from build123d import *

# Parameters (mm, degrees)
SKETCH2_W           = 889
SKETCH2_H           = 860.425
SKETCH2_W_2         = 698.5
SKETCH2_H_2         = 685.8
BOSS_EXTRUDE1_DEPTH = 114.3
SKETCH3_W           = 82.55
SKETCH3_H           = 79.375
CUT_EXTRUDE1_DEPTH  = 115.3
FILLET1_R           = 6.35


with BuildPart() as part:
    # Sketch2 → Boss-Extrude1 (new body)
    with BuildSketch(Plane(origin=(0, 0, 0), x_dir=(1, 0, 0), z_dir=(0, 1, 0))):
        with Locations((0, 7.9375)):
            Rectangle(SKETCH2_W, SKETCH2_H)
        Rectangle(SKETCH2_W_2, SKETCH2_H_2, mode=Mode.SUBTRACT)
    extrude(amount=BOSS_EXTRUDE1_DEPTH)

    # Sketch3 → Cut-Extrude1 (cut, through all)
    with BuildSketch(Plane(origin=(0, 114.3, 0), x_dir=(1, 0, 0), z_dir=(0, 1, 0))):
        with Locations((168.275, -382.5875)):
            Rectangle(SKETCH3_W, SKETCH3_H)
    extrude(amount=-CUT_EXTRUDE1_DEPTH, mode=Mode.SUBTRACT)

    # Fillet1
    fillet1_edges = [part.edges().sort_by_distance(p)[0] for p in [
        (444.5, 114.3, -7.9375),
        (0, 114.3, -438.15),
        (327.025, 0, 422.275),
        (327.025, 114.3, 422.275),
        (-444.5, 114.3, -7.9375),
        (0, 0, -438.15),
        (444.5, 0, -7.9375),
        (-158.75, 0, 422.275),
        (-444.5, 0, -7.9375),
        (-444.5, 57.15, -438.15),
        (444.5, 57.15, -438.15),
        (444.5, 57.15, 422.275),
        (-444.5, 57.15, 422.275),
        (-158.75, 114.3, 422.275),
    ]]
    fillet(fillet1_edges, radius=FILLET1_R)


solid = part.part
Check sheet for the modelled part. Datum: model origin and axes. Units: mm. A direction names the side the tool comes from. Coordinates: 2 decimals unless noted, no trailing zeros. Write each loop counter-clockwise with the first axis right and the second up, starting at its lowest first coordinate (ties: lowest second). Pieces come first, ordered by that corner, then holes.
Item 1: Mould release check, pull along Z, two halves, no side actions. Record for faces 1 (the face through (349.25, 56, 5)), 2 (the face through (-6, 114.3, -391)), 3 (the face through (-160, 56, 422.275)), 4 (the face through (-6, 56, -438.15)): released by +Z, released by -Z, zero draft, split by the parting line, or undercut.
Numbers:
face 1: undercut
face 2: zero draft
face 3: released by +Z
face 4: released by -Z
Item 2: Access from +Z, -Z, +X, -X, +Y, -Y to the whole of each face (thin tool, end or side, straight path). Record for faces 5 (the face through (-6, 0, -391)), 6 (the face through (209.55, 58, 383)), 7 (the face through (-5, 56, -342.9)).
Numbers:
face 5: +Z, -Z, +X, -X, -Y
face 6: +Z, +Y, -Y
face 7: +Y, -Y
Item 3: Cross-section at B-B on x = -151.5. Record the boundary of the cut face in (y, z) (3 decimals).
Numbers:
outline: (0, -431.8) arc R6.35 ccw to (6.35, -438.15) - (107.95, -438.15) arc R6.35 ccw to (114.3, -431.8) - (114.3, -342.9) - (0, -342.9) - close; (0, 342.9) - (114.3, 342.9) - (114.3, 415.925) arc R6.35 ccw to (107.95, 422.275) - (6.35, 422.275) arc R6.35 ccw to (0, 415.925) - close
Item 4: Scan lines: probe 1 along X at (y, z) = (48.5, 306); probe 2 along X at (y, z) = (25, 357); probe 3 along Z at (x, y) = (-193.5, 46.5) (3 decimals). Record each from-to range of solid material in increasing order.
Numbers:
probe 1: x = -444.5 to -349.25, 349.25 to 444.5
probe 2: x = -444.5 to 127, 209.55 to 444.5
probe 3: z = -438.15 to -342.9, 342.9 to 422.275
Item 5: Cross-section at A-A on z = 327.5. Record the boundary of the cut face in (x, y).
Numbers:
outline: (-444.5, 6.35) arc R6.35 ccw to (-438.15, 0) - (-349.25, 0) - (-349.25, 114.3) - (-438.15, 114.3) arc R6.35 ccw to (-444.5, 107.95) - close; (349.25, 0) - (438.15, 0) arc R6.35 ccw to (444.5, 6.35) - (444.5, 107.95) arc R6.35 ccw to (438.15, 114.3) - (349.25, 114.3) - close
Item 6: Cross-section at C-C on y = 24.5. Record the boundary of the cut face in (x, z) (3 decimals).
Numbers:
outline: (-444.5, -431.8) arc R6.35 ccw to (-438.15, -438.15) - (438.15, -438.15) arc R6.35 ccw to (444.5, -431.8) - (444.5, 415.925) arc R6.35 ccw to (438.15, 422.275) - (209.55, 422.275) - (209.55, 342.9) - (349.25, 342.9) - (349.25, -342.9) - (-349.25, -342.9) - (-349.25, 342.9) - (127, 342.9) - (127, 422.275) - (-438.15, 422.275) arc R6.35 ccw to (-444.5, 415.925) - close
